Model file for the job. Use its own axes, mm. A direction names the side the tool comes from. Coordinates: 2 decimals unless noted, no trailing zeros. Loops run counter-clockwise (first coordinate to the right, second up) from the corner with the lowest first, then second, coordinate; pieces in that order, holes last. Notation, with made-up numbers: (9.25, -25.5) -> (39.25, -25.5) arc R3 cw to (39.25, -20.5) -> close; hole circle Ø3 at (84, -32). An arc over 180 degrees is marked (long way). Use one line per item in the form item = value.
```python
from build123d import *

# Parameters (mm, degrees)
F0_W     = 4
F0_H     = 38.3
F0_R     = 1.75
F0_R_2   = 11.25
F1_DEPTH = 4
F3_DEPTH = 20
F4_R     = 2.75
F5_DEPTH = 4
F6_R     = 2.5
F7_W     = 0.5
F7_H     = 4
F8_DEPTH = 1


with BuildPart() as f1:
    # F0 (on Top) → F1 (new body)
    with BuildSketch(Plane.XY):
        with Locations((-23.15, 2)):
            Rectangle(F0_W, F0_H)
        Polygon((21.15, 21.15), (-21.15, 21.15), (-21.15, -17.15), (-21.15, -21.15), (21.15, -21.15), (21.15, -17.15), align=None)
        with Locations((-15.495, -15.495)):
            Circle(F0_R, mode=Mode.SUBTRACT)
        with Locations((15.495, -15.495)):
            Circle(F0_R, mode=Mode.SUBTRACT)
        with Locations((-15.495, 15.495)):
            Circle(F0_R, mode=Mode.SUBTRACT)
        Circle(F0_R_2, mode=Mode.SUBTRACT)
        with Locations((15.495, 15.495)):
            Circle(F0_R, mode=Mode.SUBTRACT)
        with Locations((23.15, 2)):
            Rectangle(F0_W, F0_H)
        Polygon((-21.15, -21.15), (-21.15, -17.15), (-25.15, -17.15), (-40.15, -17.15), (-40.15, -21.15), align=None)
        Polygon((25.15, -17.15), (21.15, -17.15), (21.15, -21.15), (40.15, -21.15), (40.15, -17.15), align=None)
    extrude(amount=F1_DEPTH)

    # F2 (on face) → F3 (join)
    with BuildSketch(Plane(origin=(0, 0, 0), x_dir=(1, 0, 0), z_dir=(0, 0, -1))):
        Polygon((-25.15, -21.15), (-21.15, -21.15), (-21.15, 17.15), (-21.15, 21.15), (-40.15, 21.15), (-40.15, 17.15), (-25.15, 17.15), align=None)
        Polygon((21.15, 17.15), (21.15, -21.15), (25.15, -21.15), (25.15, 17.15), (40.15, 17.15), (40.15, 21.15), (21.15, 21.15), align=None)
    extrude(amount=F3_DEPTH)

    # F4 (on face) → F5 (cut, through all)
    with BuildSketch(Plane.XZ.offset(21.15)):
        with Locations((-32.65, -10)):
            Circle(F4_R)
        with Locations((32.65, -10)):
            Circle(F4_R)
    extrude(amount=-F5_DEPTH, mode=Mode.SUBTRACT)

    # F6
    f6_edges = [f1.edges().sort_by_distance(p)[0] for p in [
        (-40.15, -19.15, 4),
        (-40.15, -19.15, -20),
        (40.15, -19.15, -20),
        (40.15, -19.15, 4),
        (25.15, -17.15, -8),
        (-25.15, -17.15, -8),
        (21.15, -21.15, -10),
        (-21.15, -21.15, -10),
    ]]
    fillet(f6_edges, radius=F6_R)

    # F7 (on face) → F8 (cut)
    with BuildSketch(Plane.XZ.offset(21.15)):
        with Locations((0.25, 2)):
            Rectangle(F7_W, F7_H)
        with Locations((-0.25, 2)):
            Rectangle(F7_W, F7_H)
    extrude(amount=-F8_DEPTH, mode=Mode.SUBTRACT)


solid = f1.part
```
Q1. Band-saw the part on B-B, the plane z = -15.5. Write the cut outline in (x, y).
Result:
outline = (-40.15, -21.15) -> (-23.65, -21.15) arc R2.5 ccw to (-21.15, -18.65) -> (-21.15, 21.15) -> (-25.15, 21.15) -> (-25.15, -14.65) arc R2.5 cw to (-27.65, -17.15) -> (-40.15, -17.15) -> close; (21.15, -18.65) arc R2.5 ccw to (23.65, -21.15) -> (40.15, -21.15) -> (40.15, -17.15) -> (27.65, -17.15) arc R2.5 cw to (25.15, -14.65) -> (25.15, 21.15) -> (21.15, 21.15) -> close
Q2. Band-saw the part on D-D, the plane y = -10. Write the cut outline in (x, z).
Result:
outline = (-25.15, -20) -> (-21.15, -20) -> (-21.15, 0) -> (-5.15, 0) -> (-5.15, 4) -> (-25.15, 4) -> close; (5.15, 0) -> (21.15, 0) -> (21.15, -20) -> (25.15, -20) -> (25.15, 4) -> (5.15, 4) -> close
Q3. Pin check, flat tips, straight feed: pin 1 Ø5 at (y, z) = (-12.5, -1) entering from -X; pin 2 Ø3 at (y, z) = (-6.5, 1) entering from -X; pin 3 Ø2 at (y, z) = (-10.5, -2) entering from +X; pin 4 Ø3 at (x, y) = (-15.495, 15.495) entering from -Z. Stop position of each tip, or through.
Result:
pin_1 = -25.17
pin_2 = -25.15
pin_3 = 25.15
pin_4 = through
Q4. Which spindle directions (+Z, -Z, +X, -X, +Y, -Y) get a long thin tool onto all of the face, cutting with end or side? Do faces 1 (the face through (-35, -17.15, -8)), 2 (the face through (-21.15, 2, -10)), 3 (the face through (40.15, -19, -8)), 4 (the face through (-40.15, -19, -8)), 5 (the face through (-21.863, -20.398, -10.14)). Say none if no direction does.
Result:
face_1 = +Z, -Z, -X, +Y
face_2 = -Z, +Y, -Y
face_3 = +Z, -Z, +X, +Y, -Y
face_4 = +Z, -Z, -X, +Y, -Y
face_5 = -Z, -Y
Q5. Mould opens along X. For faces 6 (the face through (25.863, -16.398, -8.168)), 7 (the face through (-25.15, 3, -8)), 8 (the face through (-24, -21.15, -5)), 9 (the face through (15.1, -17.2, 2)) say: released by +X, released by -X, zero draft, split by the parting line, or undercut.
Result:
face_6 = released by +X
face_7 = released by -X
face_8 = zero draft
face_9 = undercut
Q6. Wall check: line 1 along X through (y, z) = (15.5, 0.75) (3 decimals); line 2 along X through (y, z) = (2, -18); line 3 along Y through (x, z) = (0, 1.5). Give the ranges that are in metal, low to high.
Result:
line_1 = -25.15 to -17.245, -13.745 to 13.745, 17.245 to 25.15
line_2 = -25.15 to -21.15, 21.15 to 25.15
line_3 = -20.15 to -11.25, 11.25 to 21.15
Q7. Band-saw the part on C-C, the plane x = -32.65. Write the cut outline in (y, z).
Result:
outline = (-21.15, -20) -> (-17.15, -20) -> (-17.15, -12.75) -> (-21.15, -12.75) -> close; (-21.15, -7.25) -> (-17.15, -7.25) -> (-17.15, 4) -> (-21.15, 4) -> close
Q8. Band-saw the part on A-A, the plane z = -10. Write the cut outline in (x, y).
Result:
outline = (-40.15, -21.15) -> (-35.4, -21.15) -> (-35.4, -17.15) -> (-40.15, -17.15) -> close; (-29.9, -21.15) -> (-23.65, -21.15) arc R2.5 ccw to (-21.15, -18.65) -> (-21.15, 21.15) -> (-25.15, 21.15) -> (-25.15, -14.65) arc R2.5 cw to (-27.65, -17.15) -> (-29.9, -17.15) -> close; (21.15, -18.65) arc R2.5 ccw to (23.65, -21.15) -> (29.9, -21.15) -> (29.9, -17.15) -> (27.65, -17.15) arc R2.5 cw to (25.15, -14.65) -> (25.15, 21.15) -> (21.15, 21.15) -> close; (35.4, -21.15) -> (40.15, -21.15) -> (40.15, -17.15) -> (35.4, -17.15) -> close
